from build123d import *

# Parameters (mm, degrees)
SKETCH1_W           = 225.425
SKETCH1_H           = 304.8
BOSS_EXTRUDE1_DEPTH = 12.7
CUT_EXTRUDE1_DEPTH  = 9.525
CHAMFER2_SIZE       = 4.7625
CHAMFER1_SIZE       = 3.175


with BuildPart() as part:
    # Sketch1 → Boss-Extrude1 (new body)
    with BuildSketch(Plane.XY):
        Rectangle(SKETCH1_W, SKETCH1_H)
    extrude(amount=BOSS_EXTRUDE1_DEPTH)

    # Sketch2 → Cut-Extrude1 (cut)
    with BuildSketch(Plane.XY.offset(12.7)):
        with BuildLine():
            Line((96.3625, -142.4), (-96.3625, -142.4))
            ThreePointArc((-96.3625, -142.4), (-100.852628061, -140.540128061), (-102.7125, -136.05))
            Line((-102.7125, -136.05), (-102.7125, 136.05))
            ThreePointArc((-102.7125, 136.05), (-100.852628061, 140.540128061), (-96.3625, 142.4))
            Line((-96.3625, 142.4), (96.3625, 142.4))
            ThreePointArc((96.3625, 142.4), (100.852628061, 140.540128061), (102.7125, 136.05))
            Line((102.7125, 136.05), (102.7125, -136.05))
            ThreePointArc((102.7125, -136.05), (100.852628061, -140.540128061), (96.3625, -142.4))
        make_face()
    extrude(amount=-CUT_EXTRUDE1_DEPTH, mode=Mode.SUBTRACT)

    # Chamfer2
    chamfer2_edges = [part.edges().sort_by_distance(p)[0] for p in [
        (-112.7125, 152.4, 6.35),
        (112.7125, 152.4, 6.35),
        (112.7125, -152.4, 6.35),
        (-112.7125, -152.4, 6.35),
    ]]
    chamfer(chamfer2_edges, length=CHAMFER2_SIZE)

    # Chamfer1
    chamfer1_edges = [part.edges().sort_by_distance(p)[0] for p in [
        (0, -152.4, 12.7),
        (-112.7125, 0, 12.7),
        (112.7125, 0, 12.7),
        (0, 152.4, 12.7),
        (110.33125, 150.01875, 12.7),
        (110.33125, -150.01875, 12.7),
        (-110.33125, 150.01875, 12.7),
        (-110.33125, -150.01875, 12.7),
    ]]
    chamfer(chamfer1_edges, length=CHAMFER1_SIZE)


solid = part.part
Here's how the part is built. I have some questions about the finished solid (model axes, mm). A direction names the side the tool comes from. Give positions to 0.01 mm unless a question says otherwise; leave off trailing zeros. Order: outer loops, then holes, each group sorted by start corner. A loop starts at its lowest first (then second) coordinate and runs counter-clockwise, first axis right, second up. Notation, with made-up numbers: M -25.75,26.25 L 23.25,26.25 A20 cw 23.25,33.25 Z; hole C 22,-31.5 d9. An arc over 180 degrees is marked long. Answer as a JSON object with one key per item and string values. Group by question number.
1) Please list where these lines run through material, in increasing order: L1, parallel to X at y = 130.5, z = 7.75; L2, parallel to Y at x = -46, z = 7.25; L3, parallel to Z at x = 69, y = 108.5 (3 decimals). Write a range as [from, to].
2) Suppose I cut it at B-B, the plane x = -83.5. Write out the boundary of the cut face in (y, z) (3 decimals).
3) We'd pull the mould along Y, two halves only. Please class faces 3 (the flat face through (-109.23, 148.85, 11.13)), 4 (the flat face through (-112.712, -2, 5)), 5 (the flat face through (1, -142.4, 8)): pulls with the +Y half, pulls with the -Y half, needs draft (parallel to the pull), parting line crosses it, or undercut.
4) Suppose I cut it at A-A, the plane z = 6. Write out the boundary of the cut face in (x, y).
5) I'm going to push a flat-ended pin straight in: pin 1 Ø1 at (x, z) = (-3, 10.5) entering from +Y (3 decimals). Where does the tip first touch, or does it pass through?
6) On a 3-axis mill with a long thin cutter (end or side, diameter ignored), from which of +Z, -Z, +X, -X, +Y, -Y can I reach the whole of each face in a straight line? I mean faces 1 (the flat face through (-109.23, -148.85, 11.13)), 2 (the flat face through (-102.712, -2, 8)). Say none if no direction works.
7) Suppose I cut it at C-C, the plane y = 69. Write out the boundary of the cut face in (x, z) (1 decimal).
Results found:
{
 "1": {"L1": "[-112.71, -102.71], [102.71, 112.71]", "L2": "[-152.4, -142.4], [142.4, 152.4]", "L3": "[0, 3.175]"},
 "2": {"outline": "M -152.4,0 L 152.4,0 L 152.4,9.525 L 149.225,12.7 L 142.4,12.7 L 142.4,3.175 L -142.4,3.175 L -142.4,12.7 L -149.225,12.7 L -152.4,9.525 Z"},
 "3": {"face 3": "pulls with the +Y half", "face 4": "needs draft", "face 5": "undercut"},
 "4": {"outline": "M -112.71,-147.64 L -107.95,-152.4 L 107.95,-152.4 L 112.71,-147.64 L 112.71,147.64 L 107.95,152.4 L -107.95,152.4 L -112.71,147.64 Z; hole M -102.71,-136.05 A6.35 ccw -96.36,-142.4 L 96.36,-142.4 A6.35 ccw 102.71,-136.05 L 102.71,136.05 A6.35 ccw 96.36,142.4 L -96.36,142.4 A6.35 ccw -102.71,136.05 Z"},
 "5": {"pin 1": "y = 151.925"},
 "6": {"face 1": "+Z, -X, -Y", "face 2": "+Z"},
 "7": {"outline": "M -112.7,0 L 112.7,0 L 112.7,9.5 L 109.5,12.7 L 102.7,12.7 L 102.7,3.2 L -102.7,3.2 L -102.7,12.7 L -109.5,12.7 L -112.7,9.5 Z"}
}
